Here's the drawing with two shaded views (mm, measured from the low corner). I have some questions. Coordinates: 2 decimals unless noted, no trailing zeros. Order: outer loops, then holes, each group sorted by start corner. A loop starts at its lowest first (then second) coordinate and runs counter-clockwise, first axis right, second up. Notation, with made-up numbers: (5, 87.25) - (32, 87.25) arc R26 ccw to (32, 117.25) - close; hole circle Ø3 at (78.5, 55.5). An arc over 180 degrees is marked (long way). Answer as CSV lines item,"result". Start each with the question number.
1. I want a section at B-B, the plane x = 25. List the corners of the cut face in (y, z) for me, and give its area (3 significant figures).
2. I want a section at D-D, the plane x = 13. List the corners of the cut face in (y, z) for me.
3. I need wall thicknesses on probe 1 along X at (y, z) = (0.3, 4); probe 2 along X at (y, z) = (0.65, 20); probe 3 along Z at (x, y) = (25.5, 0.8). Which ranges of each line are inside material? Lowest first, please.
4. I want a section at C-C, the plane y = 1.05. List the corners of the cut face in (x, z) for me.
5. For pin 1 (0.8 mm diameter, centred on x = 2.5, y = 0.5, fed in from -Z); pin 2 (0.8 mm diameter, centred on y = 0.5, z = 4, fed in from -X), each with a flat end and sliding along its axis, tell me the tip position at first contact or that it passes through.
6. I want a section at A-A, the plane z = 4. List the corners of the cut face in (x, y) for me, and give its area (3 significant figures).
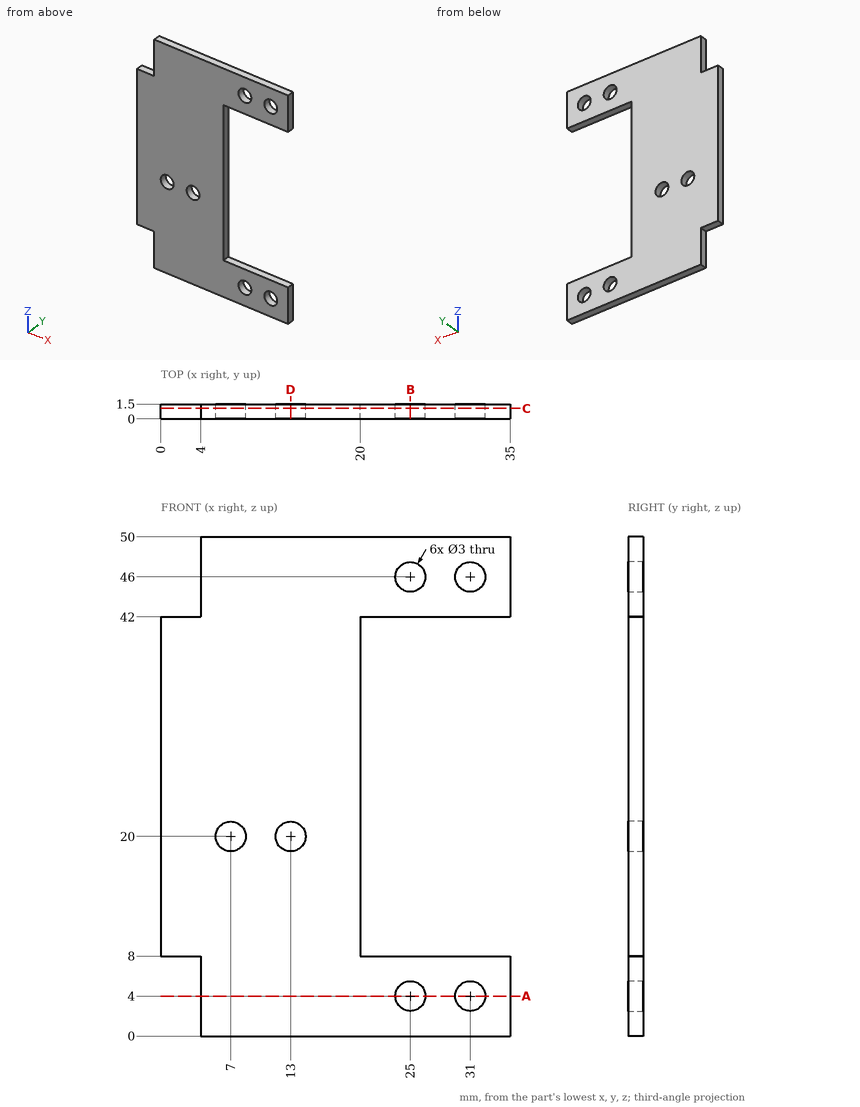
Solved:
1,outline,"(0, 0) - (1.5, 0) - (1.5, 2.5) - (0, 2.5) - close; (0, 5.5) - (1.5, 5.5) - (1.5, 8) - (0, 8) - close; (0, 42) - (1.5, 42) - (1.5, 44.5) - (0, 44.5) - close; (0, 47.5) - (1.5, 47.5) - (1.5, 50) - (0, 50) - close"
1,area,"15.0 mm2"
2,outline,"(0, 0) - (1.5, 0) - (1.5, 18.5) - (0, 18.5) - close; (0, 21.5) - (1.5, 21.5) - (1.5, 50) - (0, 50) - close"
3,probe 1,"x = 4 to 23.5, 26.5 to 29.5, 32.5 to 35"
3,probe 2,"x = 0 to 5.5, 8.5 to 11.5, 14.5 to 20"
3,probe 3,"z = 0 to 2.59, 5.41 to 8, 42 to 44.59, 47.41 to 50"
4,outline,"(0, 8) - (4, 8) - (4, 0) - (35, 0) - (35, 8) - (20, 8) - (20, 42) - (35, 42) - (35, 50) - (4, 50) - (4, 42) - (0, 42) - close; hole circle Ø3 at (7, 20); hole circle Ø3 at (13, 20); hole circle Ø3 at (25, 4); hole circle Ø3 at (25, 46); hole circle Ø3 at (31, 4); hole circle Ø3 at (31, 46)"
5,pin 1,"stops at z = 8"
5,pin 2,"stops at x = 4"
6,outline,"(4, 0) - (23.5, 0) - (23.5, 1.5) - (4, 1.5) - close; (26.5, 0) - (29.5, 0) - (29.5, 1.5) - (26.5, 1.5) - close; (32.5, 0) - (35, 0) - (35, 1.5) - (32.5, 1.5) - close"
6,area,"37.5 mm2"
